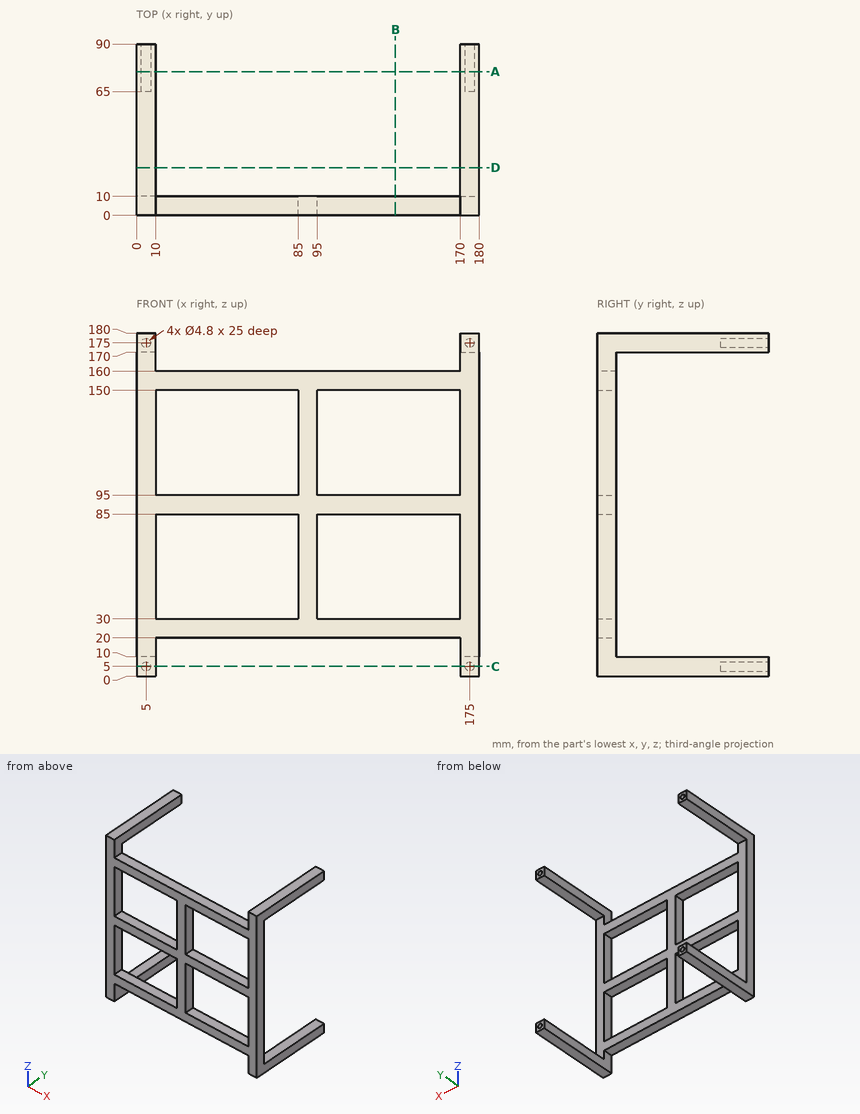
Check sheet for the drawn part. Datum: minimum x, y, z corner. Units: mm. Coordinates: 2 decimals unless noted, no trailing zeros. Write each loop counter-clockwise with the first axis right and the second up, starting at its lowest first coordinate (ties: lowest second). Pieces come first, ordered by that corner, then holes. Notation, with made-up numbers: M 61.25,37 L 108.25,37 A17 cw 108.25,48 Z; hole C 80,7 d7. An arc over 180 degrees is marked long. Use a Markdown table: item, result.
Q1. Thickness scan on line 1 (Z direction, x = 5, y = 78); line 2 (Y direction, x = 133.5, z = 158). Record the ranges inside material, lowest first.
Reply:
| item | result |
|---|---|
| line 1 | z = 0 to 2.6, 7.4 to 10, 170 to 172.6, 177.4 to 180 |
| line 2 | y = 0 to 10 |
Q2. Sectioned sample at D-D, the plane y = 25. Record the boundary of the cut face in (x, z), plus the area to 3 significant figures.
Reply:
| item | result |
|---|---|
| outline | M 0,0 L 10,0 L 10,10 L 0,10 Z; M 0,170 L 10,170 L 10,180 L 0,180 Z; M 170,0 L 180,0 L 180,10 L 170,10 Z; M 170,170 L 180,170 L 180,180 L 170,180 Z |
| area | 400 mm² |
Q3. Sectioned sample at A-A, the plane y = 75.5. Record the boundary of the cut face in (x, z), plus the area to 3 significant figures.
Reply:
| item | result |
|---|---|
| outline | M 0,0 L 10,0 L 10,10 L 0,10 Z; M 0,170 L 10,170 L 10,180 L 0,180 Z; M 170,0 L 180,0 L 180,10 L 170,10 Z; M 170,170 L 180,170 L 180,180 L 170,180 Z; hole C 5,5 d4.8; hole C 5,175 d4.8; hole C 175,5 d4.8; hole C 175,175 d4.8 |
| area | 328 mm² |
Q4. Sectioned sample at C-C, the plane z = 5. Record the boundary of the cut face in (x, y).
Reply:
| item | result |
|---|---|
| outline | M 0,0 L 10,0 L 10,90 L 7.4,90 L 7.4,65 L 2.6,65 L 2.6,90 L 0,90 Z; M 170,0 L 180,0 L 180,90 L 177.4,90 L 177.4,65 L 172.6,65 L 172.6,90 L 170,90 Z |
Q5. Go/stop test with flat-tipped pins: P1, Ø3, axis at x = 5, y = 65.5, coming from the -Z side; P2, Ø11, axis at x = 58, y = 7, coming from the -Z side; P3, Ø6, axis at y = 31.5, z = 165.5, coming from the +X side; P4, Ø1.4, axis at x = 176, z = 5.5, coming from the +Y side. Record where each tip stops, or that it passes through.
Reply:
| item | result |
|---|---|
| P1 | stops at z = 0 |
| P2 | stops at z = 20 |
| P3 | passes through |
| P4 | stops at y = 65 |
Q6. Sectioned sample at B-B, the plane x = 136. Record the boundary of the cut face in (y, z).
Reply:
| item | result |
|---|---|
| outline | M 0,20 L 10,20 L 10,30 L 0,30 Z; M 0,85 L 10,85 L 10,95 L 0,95 Z; M 0,150 L 10,150 L 10,160 L 0,160 Z |
